Print and shaded views of the part. All mm, measured from the part's lowest x, y and z. Give positions to 0.01 mm unless a question says otherwise; leave off trailing zeros. Loops run counter-clockwise (first coordinate to the right, second up) from the corner with the lowest first, then second, coordinate; pieces in that order, holes last. Notation, with made-up numbers: M 20.25,68 L 34.25,68 A18 ccw 34.25,88 Z; hole C 79.25,39 d5. An arc over 180 degrees is marked long. Answer as CSV lines item,"result".
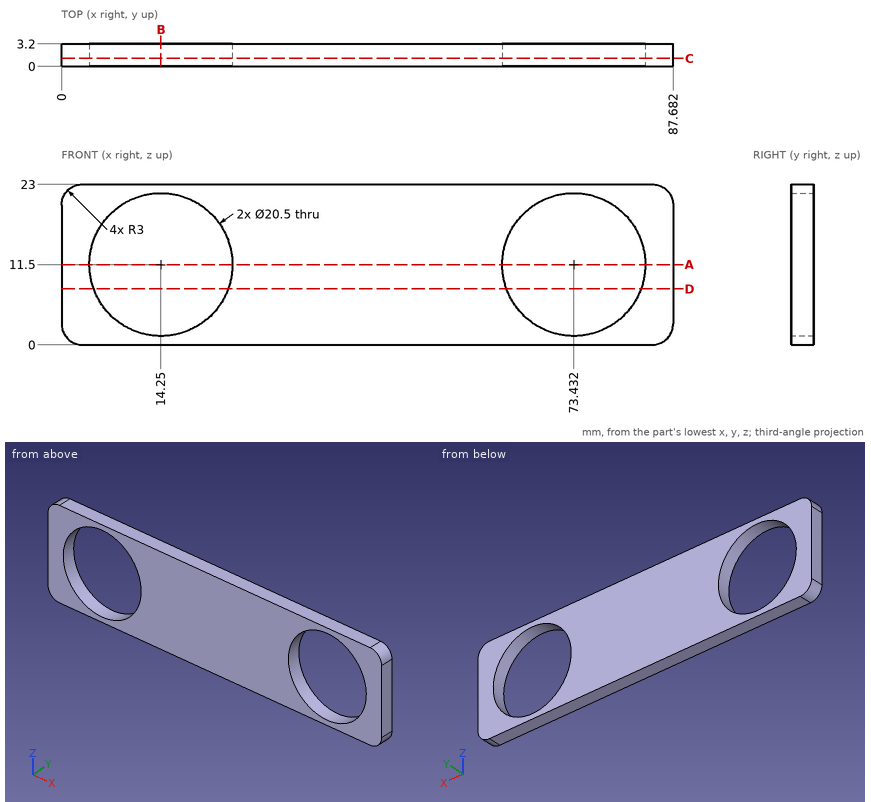
Q1. Wall check: line 1 (X direction, y = 2.1, z = 11.75); line 2 (X direction, y = 2.45, z = 9.5); line 3 (Z direction, x = 11.5, y = 2.9). Give the ranges that are in metal, low to high. Write a range as [from, to].
Solution:
line 1,"x = [0, 4], [24.5, 63.19], [83.68, 87.68]"
line 2,"x = [0, 4.2], [24.3, 63.38], [83.48, 87.68]"
line 3,"z = [0, 1.63], [21.37, 23]"
Q2. Cut at D-D (z = 8). Write the cut outline in (x, y), and give its area (3 significant figures).
Solution:
outline,"M 0,0 L 4.62,0 L 4.62,3.2 L 0,3.2 Z; M 23.88,0 L 63.8,0 L 63.8,3.2 L 23.88,3.2 Z; M 83.07,0 L 87.68,0 L 87.68,3.2 L 83.07,3.2 Z"
area,"157 mm²"
Q3. Cut at B-B (x = 14.25). Write the cut outline in (y, z), and give its area (3 significant figures).
Solution:
outline,"M 0,0 L 3.2,0 L 3.2,1.25 L 0,1.25 Z; M 0,21.75 L 3.2,21.75 L 3.2,23 L 0,23 Z"
area,"8.00 mm²"
Q4. Cut at C-C (y = 1.15). Write the cut outline in (x, z), and give its area (3 significant figures).
Solution:
outline,"M 0,3 A3 ccw 3,0 L 84.68,0 A3 ccw 87.68,3 L 87.68,20 A3 ccw 84.68,23 L 3,23 A3 ccw 0,20 Z; hole C 14.25,11.5 d20.5; hole C 73.43,11.5 d20.5"
area,"1,350 mm²"
Q5. Cut at A-A (z = 11.5). Write the cut outline in (x, y), and give its area (3 significant figures).
Solution:
outline,"M 0,0 L 4,0 L 4,3.2 L 0,3.2 Z; M 24.5,0 L 63.18,0 L 63.18,3.2 L 24.5,3.2 Z; M 83.68,0 L 87.68,0 L 87.68,3.2 L 83.68,3.2 Z"
area,"149 mm²"
